Part print with two shaded views. Sizes in mm from the minimum x, y, z corner. Coordinates: 2 decimals unless noted, no trailing zeros. Loops run counter-clockwise (first coordinate to the right, second up) from the corner with the lowest first, then second, coordinate; pieces in that order, holes last.
(1) Slice it at B-B (y = 4.75). Give the cut face in (x, z), and give its area (3 significant figures).
(2) Slice it at A-A (y = 23.5). Give the cut face in (x, z), and give its area (3 significant figures).
(3) Slice it at C-C (x = 16). Give the cut face in (y, z), and give its area (3 significant figures).
(4) Flat gauge pin, fed straight in: P1, Ø4, axis at x = 42.25, y = 23.5, coming from the -Z side. Where does the tip first touch, or does it go through?
(5) Wall check: L1, parallel to Y at x = 23.5, z = 0.6; L2, parallel to Y at x = 16, z = 0.7. Give the ranges that are in metal, low to high.
(6) Slice it at D-D (z = 0.15). Give the cut face in (x, y).
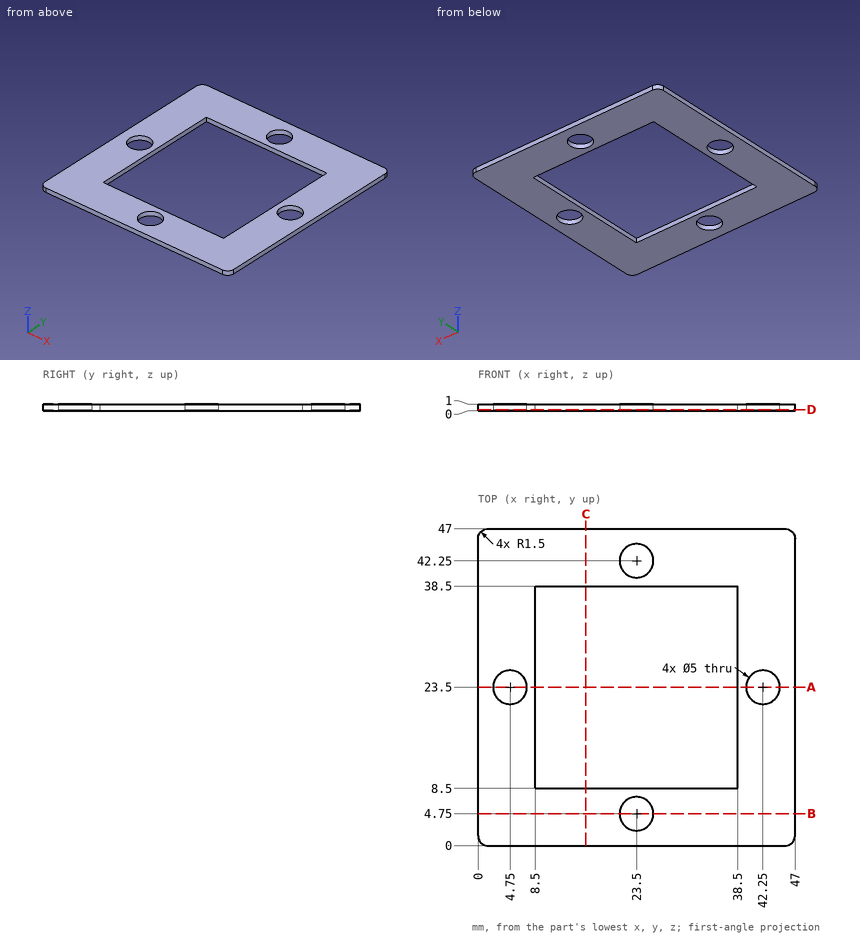
Response values:
1. outline: (0, 0) - (21, 0) - (21, 1) - (0, 1) - close; (26, 0) - (47, 0) - (47, 1) - (26, 1) - close
1. area: 42.0 mm2
2. outline: (0, 0) - (2.25, 0) - (2.25, 1) - (0, 1) - close; (7.25, 0) - (8.5, 0) - (8.5, 1) - (7.25, 1) - close; (38.5, 0) - (39.75, 0) - (39.75, 1) - (38.5, 1) - close; (44.75, 0) - (47, 0) - (47, 1) - (44.75, 1) - close
2. area: 7.00 mm2
3. outline: (0, 0) - (8.5, 0) - (8.5, 1) - (0, 1) - close; (38.5, 0) - (47, 0) - (47, 1) - (38.5, 1) - close
3. area: 17.0 mm2
4. P1: passes through
5. L1: y = 0 to 2.25, 7.25 to 8.5, 38.5 to 39.75, 44.75 to 47
5. L2: y = 0 to 8.5, 38.5 to 47
6. outline: (0, 1.5) arc R1.5 ccw to (1.5, 0) - (45.5, 0) arc R1.5 ccw to (47, 1.5) - (47, 45.5) arc R1.5 ccw to (45.5, 47) - (1.5, 47) arc R1.5 ccw to (0, 45.5) - close; hole circle Ø5 at (4.75, 23.5); hole (8.5, 8.5) - (38.5, 8.5) - (38.5, 38.5) - (8.5, 38.5) - close; hole circle Ø5 at (23.5, 4.75); hole circle Ø5 at (23.5, 42.25); hole circle Ø5 at (42.25, 23.5)
